For this review, take the finished solid that the model builds, in its own axes (mm). Face numbers are marked on the shaded views. A direction names the side the tool comes from. Coordinates: 2 decimals unless noted, no trailing zeros. Order: outer loops, then holes, each group sorted by start corner. A loop starts at its lowest first (then second) coordinate and runs counter-clockwise, first axis right, second up.
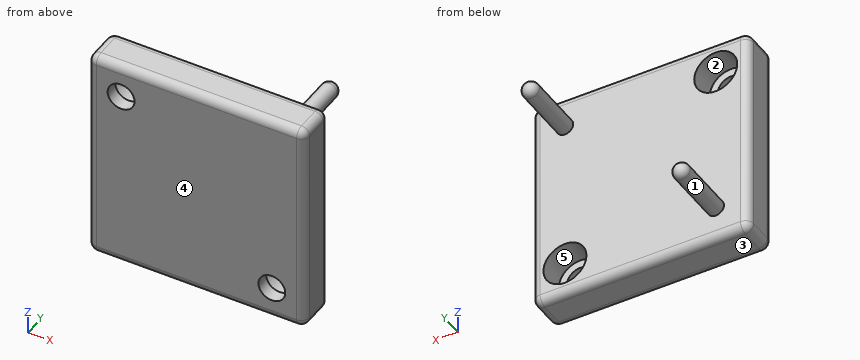
Autodesk Inventor part; units mm, degrees
ref_plane "YZ Plane" through (0, 0, 0) normal (1, 0, 0) x (0, 1, 0)
ref_plane "XZ Plane" through (0, 0, 0) normal (0, 1, 0) x (-1, 0, 0)
ref_plane "XY Plane" through (0, 0, 0) normal (0, 0, 1) x (1, 0, 0)
sketch "Sketch1" plane through (0, 0, 0) normal (0, 1, 0) x (-1, 0, 0)
  circle A0 centre (19.5118, 57.0521) radius 2.5797
  circle A1 centre (19.5118, 28.0961) radius 1.5875
  circle A2 centre (-9.4442, 28.0961) radius 2.5797
  circle A3 centre (-9.4442, 57.0521) radius 1.5875
  line L0 (25.8618, 63.4021) -> (-15.7942, 63.4021)
  line L1 (-15.7942, 63.4021) -> (-15.7942, 21.7461)
  line L2 (-15.7942, 21.7461) -> (25.8618, 21.7461)
  line L3 (25.8618, 21.7461) -> (25.8618, 63.4021)
  point P0 (0, 0)
  dimension "d0" = 5.1594
  dimension "d1" = 3.175
  dimension "d2" = 28.956
  dimension "d3" = 5.1594
  dimension "d4" = 3.175
  dimension "d5" = 28.956
  dimension "d6" = 28.956
  dimension "d7" = 28.956
  dimension "d8" = 41.656
  dimension "d9" = 41.656
  dimension "d10" = 6.35
  dimension "d11" = 6.35
extrude "Extrusion1" add sketch "Sketch1" along normal blind 7.62
sketch "Sketch2" plane through (0, 7.62, 0) normal (0, 1, 0) x (1, 0, 0)
  circle A0 centre (-19.5118, -57.0521) radius 2.5797
  circle A1 centre (-19.5118, -57.0521) radius 4.1275
  circle A2 centre (9.4442, -28.0961) radius 2.5797
  circle A3 centre (9.4442, -28.0961) radius 4.1275
  point P0 (0, 0)
  dimension "d14" = 8.255
  dimension "d15" = 8.255
extrude "Extrusion2" cut sketch "Sketch2" against normal blind 5.08 contours A0 | A1 | A2 | A3
sketch "Sketch3" plane through (0, 0, 0) normal (0, -1, 0) x (1, 0, 0)
  circle A0 centre (-19.5118, 28.0961) radius 1.5875
  circle A1 centre (-19.5118, 28.0961) radius 1.5875
  circle A2 centre (9.4442, 57.0521) radius 1.5875
  circle A3 centre (9.4442, 57.0521) radius 1.5875
  point P0 (0, 0)
extrude "Extrusion3" add sketch "Sketch3" against normal blind 20.32
fillet "Fillet1" radius 1.5875 8 edges at (-25.8618, 7.62, 42.5741) (-5.0338, 7.62, 21.7461) (15.7942, 7.62, 42.5741) (-5.0338, 7.62, 63.4021) (-5.0338, 0, 63.4021) (-25.8618, 0, 42.5741) (-5.0338, 0, 21.7461) (15.7942, 0, 42.5741)
fillet "Fillet2" radius 1.5875 2 edges at (7.8567, 20.32, 57.0521) (-21.0993, 20.32, 28.0961)
fillet "Fillet3" radius 1.5875 12 edges at (15.3292, 7.155, 62.9372) (15.3292, 0.465, 62.9372) (15.7942, 3.81, 63.4021) (15.3292, 7.155, 22.2111) (15.3292, 0.465, 22.2111) (15.7942, 3.81, 21.7461) (-25.3968, 7.155, 22.2111) (-25.3968, 0.465, 22.2111) (-25.8618, 3.81, 21.7461) (-25.3968, 7.155, 62.9372) (-25.3968, 0.465, 62.9372) (-25.8618, 3.81, 63.4021)
properties part number "pigeon Mount"
1. Take a section at A-A, the plane x = -7. Give the boundary of the cut face in (y, z) (1 decimal), plus the area to 3 significant figures.
Answer below:
outline: (0, 23.3) arc R1.6 ccw to (1.6, 21.7) - (6, 21.7) arc R1.6 ccw to (7.6, 23.3) - (7.6, 61.8) arc R1.6 ccw to (6, 63.4) - (1.6, 63.4) arc R1.6 ccw to (0, 61.8) - close
area: 315 mm2
2. Clearance check with flat-ended pins moving along their axes: pin 1 Ø6.5 at (x, z) = (-19.51, 57.05) entering from +Y; pin 2 Ø3 at (x, z) = (-15.5, 27.5) entering from +Y. State where each tip first meets the part, or that it passes through.
Answer below:
pin 1: stops at y = 2.54
pin 2: stops at y = 7.62
3. Take a section at C-C, the plane x = 8.5. Give the boundary of the cut face in (y, z) (1 decimal).
Answer below:
outline: (0, 23.3) arc R1.6 ccw to (1.6, 21.7) - (6, 21.7) arc R1.6 ccw to (7.6, 23.3) - (7.6, 24.1) - (2.5, 24.1) - (2.5, 25.7) - (0, 25.7) - close; (0, 30.5) - (2.5, 30.5) - (2.5, 32.1) - (7.6, 32.1) - (7.6, 55.8) - (18.7, 55.8) arc R1.3 ccw to (18.7, 58.3) - (7.6, 58.3) - (7.6, 61.8) arc R1.6 ccw to (6, 63.4) - (1.6, 63.4) arc R1.6 ccw to (0, 61.8) - close
4. Take a section at B-B, the plane z = 33. Give the boundary of the cut face in (x, y) (1 decimal).
Answer below:
outline: (-25.9, 1.6) arc R1.6 ccw to (-24.3, 0) - (14.2, 0) arc R1.6 ccw to (15.8, 1.6) - (15.8, 6) arc R1.6 ccw to (14.2, 7.6) - (-24.3, 7.6) arc R1.6 ccw to (-25.9, 6) - close
5. Machinability: for the marked faces 4 and 5, which of the approach directions +Z, -Z, +X, -X, +Y, -Y give a long, thin tool a straight path to every point of the face, cutting with its end or side? Answer none if there is none.
Answer below:
face 4: +Z, -Z, +X, -X, -Y
face 5: +Y
6. To check wall thickness, follow L1, parallel to X at y = 1.5, z = 26; L2, parallel to Y at x = -18, z = 47.5; L3, parallel to X at y = 6.75, z = 25. State the ranges of each line that lie inside material, in increasing order.
Answer below:
L1: x = -25.86 to 7.94, 10.95 to 15.79
L2: y = 0 to 7.62
L3: x = -25.69 to 6.71, 12.17 to 15.62
7. The part is to be moulded in two halves that separate along X. For the marked faces 1, 2 and 3, say which applies: +X half, -X half, draft (parallel to the pull), parting line (faces both ways), or undercut.
Answer below:
face 1: parting line
face 2: undercut
face 3: draft
8. Take a section at D-D, the plane y = 5.5. Give the boundary of the cut face in (x, z) (1 decimal), plus the area to 3 significant figures.
Answer below:
outline: (-25.9, 23.3) arc R1.6 ccw to (-24.3, 21.7) - (14.2, 21.7) arc R1.6 ccw to (15.8, 23.3) - (15.8, 61.8) arc R1.6 ccw to (14.2, 63.4) - (-24.3, 63.4) arc R1.6 ccw to (-25.9, 61.8) - close; hole circle Ø8.3 at (-19.5, 57.1); hole circle Ø8.3 at (9.4, 28.1)
area: 1,630 mm2
